from build123d import *

# Parameters (mm, degrees)
SKETCH_1_W           = 25.3
SKETCH_1_H           = 10.1
EXTRUDE_1_DEPTH      = 7.9
SKETCH_3_W           = 1.74
SKETCH_3_H           = 5
CUT_EXTRUDE_2_DEPTH  = 0.2
SKETCH_2_OUTSIDE_W   = 32.972
SKETCH_2_OUTSIDE_H   = 17.772
SKETCH_2_OUTSIDE_W_2 = 2.042192643
SKETCH_2_OUTSIDE_H_2 = 0.593685633
CUT_EXTRUDE_1_DEPTH  = 2
SKETCH_4_R           = 0.225
EXTRUDE_2_DEPTH      = 5


with BuildPart() as part:
    # 草图1 → 凸台-拉伸1 (new body)
    with BuildSketch(Plane(origin=(0, 0, 0), x_dir=(1, 0, 0), z_dir=(0, 1, 0))):
        Rectangle(SKETCH_1_W, SKETCH_1_H)
    extrude(amount=EXTRUDE_1_DEPTH)

    # 草图3 → 切除-拉伸2 (cut)
    with BuildSketch(Plane(origin=(0, 7.9, 0), x_dir=(1, 0, 0), z_dir=(0, 1, 0))):
        with Locations((-1.27, 0)):
            Rectangle(SKETCH_3_W, SKETCH_3_H)
        with Locations((1.27, 0)):
            Rectangle(SKETCH_3_W, SKETCH_3_H)
        with Locations((3.81, 0)):
            Rectangle(SKETCH_3_W, SKETCH_3_H)
        with Locations((6.35, 0)):
            Rectangle(SKETCH_3_W, SKETCH_3_H)
        with Locations((8.89, 0)):
            Rectangle(SKETCH_3_W, SKETCH_3_H)
        with Locations((11.43, 0)):
            Rectangle(SKETCH_3_W, SKETCH_3_H)
        with Locations((-3.81, 0)):
            Rectangle(SKETCH_3_W, SKETCH_3_H)
        with Locations((-6.35, 0)):
            Rectangle(SKETCH_3_W, SKETCH_3_H)
        with Locations((-8.89, 0)):
            Rectangle(SKETCH_3_W, SKETCH_3_H)
        with Locations((-11.43, 0)):
            Rectangle(SKETCH_3_W, SKETCH_3_H)
    extrude(amount=-CUT_EXTRUDE_2_DEPTH, mode=Mode.SUBTRACT)

    # 草图2 outside → 切除-拉伸1 (cut)
    with BuildSketch(Plane.XZ):
        Rectangle(SKETCH_2_OUTSIDE_W, SKETCH_2_OUTSIDE_H)
        with Locations((-11.628903679, 4.753157184)):
            Rectangle(SKETCH_2_OUTSIDE_W_2, SKETCH_2_OUTSIDE_H_2, mode=Mode.SUBTRACT)
        with Locations((11.628903679, 4.753157184)):
            Rectangle(SKETCH_2_OUTSIDE_W_2, SKETCH_2_OUTSIDE_H_2, mode=Mode.SUBTRACT)
        with Locations((11.628903679, -4.753157184)):
            Rectangle(SKETCH_2_OUTSIDE_W_2, SKETCH_2_OUTSIDE_H_2, mode=Mode.SUBTRACT)
        with Locations((-11.628903679, -4.753157184)):
            Rectangle(SKETCH_2_OUTSIDE_W_2, SKETCH_2_OUTSIDE_H_2, mode=Mode.SUBTRACT)
    extrude(amount=-CUT_EXTRUDE_1_DEPTH, mode=Mode.SUBTRACT)

    # 草图4 → 凸台-拉伸2 (add)
    with BuildSketch(Plane.XZ.offset(-2)):
        with Locations(Location((-1.27, 3.7, 0), (0, 0, 270))):
            Circle(SKETCH_4_R)
        with Locations(Location((-1.27, -3.7, 0), (0, 0, 90))):
            Circle(SKETCH_4_R)
        with Locations(Location((1.27, 3.7, 0), (0, 0, 270))):
            Circle(SKETCH_4_R)
        with Locations(Location((1.27, -3.7, 0), (0, 0, 90))):
            Circle(SKETCH_4_R)
        with Locations(Location((3.81, 3.7, 0), (0, 0, 270))):
            Circle(SKETCH_4_R)
        with Locations(Location((3.81, -3.7, 0), (0, 0, 90))):
            Circle(SKETCH_4_R)
        with Locations(Location((6.35, 3.7, 0), (0, 0, 270))):
            Circle(SKETCH_4_R)
        with Locations(Location((6.35, -3.7, 0), (0, 0, 90))):
            Circle(SKETCH_4_R)
        with Locations(Location((8.89, 3.7, 0), (0, 0, 270))):
            Circle(SKETCH_4_R)
        with Locations(Location((8.89, -3.7, 0), (0, 0, 90))):
            Circle(SKETCH_4_R)
        with Locations(Location((11.43, 3.7, 0), (0, 0, 270))):
            Circle(SKETCH_4_R)
        with Locations(Location((11.43, -3.7, 0), (0, 0, 90))):
            Circle(SKETCH_4_R)
        with Locations(Location((-3.81, 3.7, 0), (0, 0, 270))):
            Circle(SKETCH_4_R)
        with Locations(Location((-3.81, -3.7, 0), (0, 0, 90))):
            Circle(SKETCH_4_R)
        with Locations(Location((-6.35, 3.7, 0), (0, 0, 270))):
            Circle(SKETCH_4_R)
        with Locations(Location((-6.35, -3.7, 0), (0, 0, 90))):
            Circle(SKETCH_4_R)
        with Locations(Location((-8.89, 3.7, 0), (0, 0, 270))):
            Circle(SKETCH_4_R)
        with Locations(Location((-8.89, -3.7, 0), (0, 0, 90))):
            Circle(SKETCH_4_R)
        with Locations(Location((-11.43, 3.7, 0), (0, 0, 270))):
            Circle(SKETCH_4_R)
        with Locations(Location((-11.43, -3.7, 0), (0, 0, 90))):
            Circle(SKETCH_4_R)
    extrude(amount=EXTRUDE_2_DEPTH)


solid = part.part
CAD build for the part. Positions are in the model's coordinates, mm. A direction names the side the tool comes from. Give positions to 0.01 mm unless a question says otherwise; leave off trailing zeros. Write each loop counter-clockwise with the first axis right and the second up, starting at its lowest first coordinate (ties: lowest second). Pieces come first, ordered by that corner, then holes. Notation, with made-up numbers: M 72.25,47 L 99.25,47 A27 ccw 99.25,71 Z; hole C 49.25,25 d6. An arc over 180 degrees is marked long. Put each result on its own line as item: value. Start each with the question number.
(1) Which spindle directions (+Z, -Z, +X, -X, +Y, -Y) get a long thin tool onto all of the face, cutting with end or side? Do faces 4 (the face through (0, 5, 5.05)), 5 (the face through (12, 1, -4.456)), 6 (the face through (1, 7.7, 0)). Say none if no direction does.
(2) Band-saw the part on A-A, the plane y = -2. Give the number of separate pieces and of enclosed holes in the cut face, and give its area (3 significant figures).
(3) Probe L1, parallel to Y at x = 8.75, z = 0.5; L2, parallel to Y at x = 7, z = -3.25. List the from-to ranges inside material, lowest first.
(4) Mould opens along Z. For faces 1 (the face through (0, 7.9, 0)), 2 (the face through (0, 5, -5.05)), 3 (the face through (-9, 7.7, 0)) say: +Z half, -Z half, draft (parallel to the pull), parting line (faces both ways), or undercut.
(5) Flat gauge pins, fed straight in: pin 1 Ø0.9 at (x, z) = (9, 0) entering from +Y; pin 2 Ø0.5 at (x, z) = (12, 4.5) entering from -Y; pin 3 Ø5 at (x, y) = (2.5, -1) entering from -Z (3 decimals). Where does each tip first touch, or does it go through?
(6) Band-saw the part on C-C, the plane x = 0. Write the cut outline in (y, z).
Response values:
1. face 4: +Z, +X, -X, +Y, -Y
1. face 5: +X, -X, -Y
1. face 6: +Y
2. separate pieces: 20
2. enclosed holes: 0
2. area: 3.18 mm2
3. L1: y = 2 to 7.7
3. L2: y = 2 to 7.9
4. face 1: draft
4. face 2: -Z half
4. face 3: undercut
5. pin 1: stops at y = 7.7
5. pin 2: stops at y = 0
5. pin 3: stops at z = -3.925
6. outline: M 2,-5.05 L 7.9,-5.05 L 7.9,5.05 L 2,5.05 Z
